Could you check a few things on this drawing? It's one solid part, dimensions in mm from its lowest x, y, z. Coordinates: 2 decimals unless noted, no trailing zeros. Order: outer loops, then holes, each group sorted by start corner. A loop starts at its lowest first (then second) coordinate and runs counter-clockwise, first axis right, second up. Notation, with made-up numbers: M 17.25,79.25 L 76.25,79.25 A12 cw 76.25,84.25 Z; hole C 6,22 d9. An arc over 180 degrees is marked long. Answer as CSV lines item,"result". Start each with the question number.
1. If we section it at A-A (y = 7.75): List the corners of the cut face in (x, z) for me, plus the area to 3 significant figures.
2. If we section it at B-B (z = 53): List the corners of the cut face in (x, y) for me.
3. I need wall thicknesses on line 1 along Z through (x, y) = (54.5, 5.75); line 2 along X through (y, z) = (11, 53); line 3 along Y through (x, z) = (54, 13.5). Which ranges of each line are inside material? Lowest first, please. Write a range as from..to.
4. Will these pins go through, and if not, where does the flat tip stop? pin 1 (1.5 mm diameter, centred on x = 16, z = 94, fed in from -Y); pin 2 (4 mm diameter, centred on x = 30, z = 53, fed in from -Y).
5. If we section it at C-C (x = 42): List the corners of the cut face in (y, z) for me, plus the area to 3 significant figures.
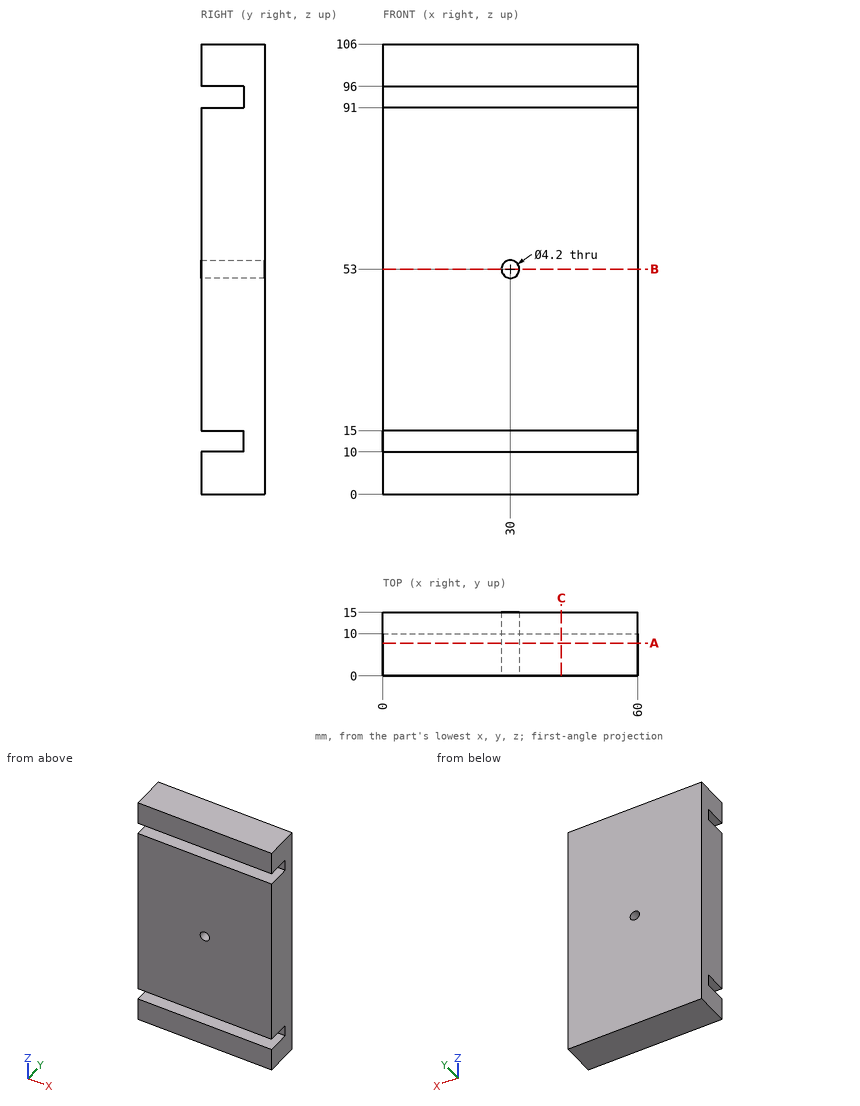
Solved:
1,outline,"M 0,0 L 60,0 L 60,10 L 0,10 Z; M 0,15 L 60,15 L 60,91 L 0,91 Z; M 0,96 L 60,96 L 60,106 L 0,106 Z; hole C 30,53 d4.2"
1,area,"5,750 mm²"
2,outline,"M 0,0 L 27.9,0 L 27.9,15 L 0,15 Z; M 32.1,0 L 60,0 L 60,15 L 32.1,15 Z"
3,line 1,"0..10, 15..91, 96..106"
3,line 2,"0..27.9, 32.1..60"
3,line 3,"10..15"
4,pin 1,"y = 10"
4,pin 2,"through"
5,outline,"M 0,0 L 15,0 L 15,106 L 0,106 L 0,96 L 10,96 L 10,91 L 0,91 L 0,15 L 10,15 L 10,10 L 0,10 Z"
5,area,"1,490 mm²"
